For this review, use the dimensioned drawing (mm, ordinates from the lowest corner) and the shaded views. A direction names the side the tool comes from. Coordinates: 2 decimals unless noted, no trailing zeros. Order: outer loops, then holes, each group sorted by start corner. A loop starts at its lowest first (then second) coordinate and runs counter-clockwise, first axis right, second up. Notation, with made-up numbers: M 44.5,-21.75 L 55.5,-21.75 A15 ccw 55.5,-9.75 Z; hole C -28.5,-24.75 d7. An arc over 180 degrees is marked long. Answer in a Markdown table with one row per item.
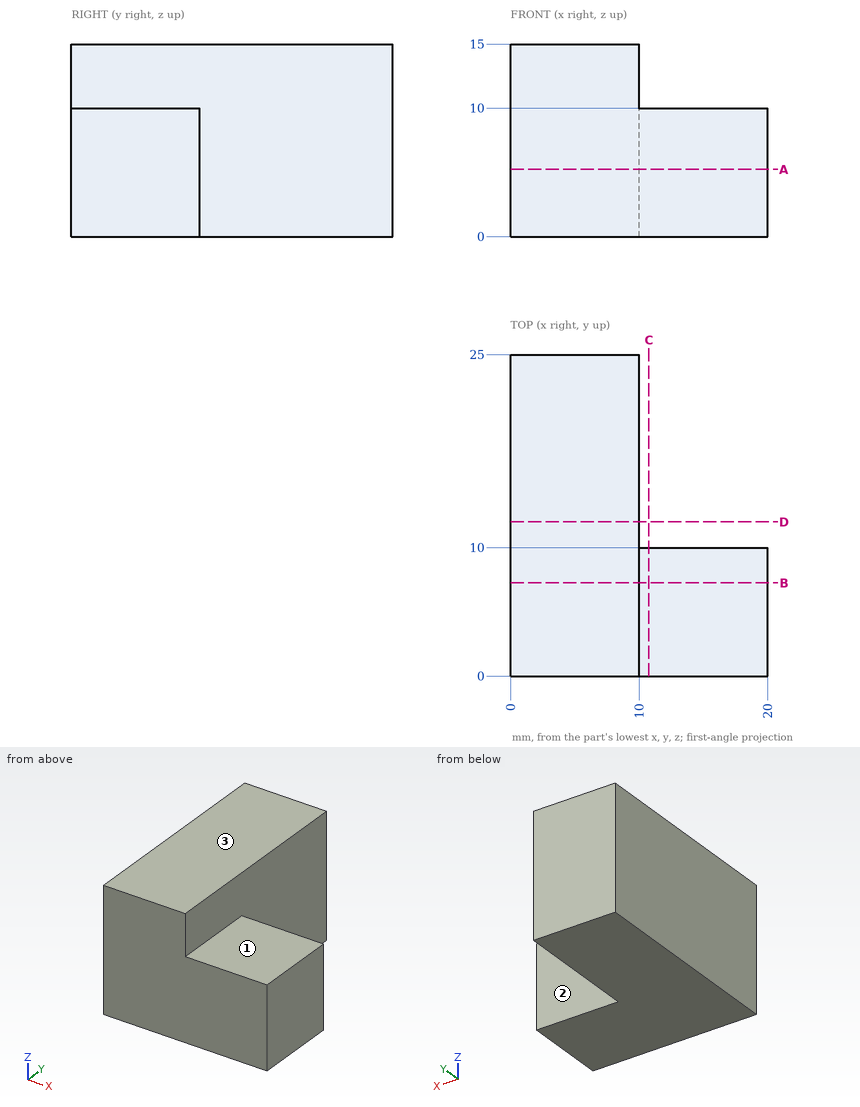
(1) Take a section at C-C (x = 10.75). Write out the cut boundary in (y, z).
Report:
| item | result |
|---|---|
| outline | M 0,0 L 10,0 L 10,10 L 0,10 Z |
(2) Take a section at D-D (y = 12). Write out the cut boundary in (x, z), then the cut area to 3 significant figures.
Report:
| item | result |
|---|---|
| outline | M 0,0 L 10,0 L 10,15 L 0,15 Z |
| area | 150 mm^2 |
(3) Take a section at A-A (z = 5.25). Write out the cut boundary in (x, y), then the cut area to 3 significant figures.
Report:
| item | result |
|---|---|
| outline | M 0,0 L 20,0 L 20,10 L 10,10 L 10,25 L 0,25 Z |
| area | 350 mm^2 |
(4) To check wall thickness, follow line 1 (X direction, y = 16.25, z = 2.25). State the ranges of the line that lie inside material, in increasing order. Write a range as [from, to].
Report:
| item | result |
|---|---|
| line 1 | [0, 10] |
(5) Insertion check: P1, Ø5, axis at x = 15, z = 8, coming from the +Y side; P2, Ø5, axis at x = 17.5, y = 5, coming from the +Z side. Each pin has a flat end and moves straight along its axis. Give the tip position at first contact, or say it passes through.
Report:
| item | result |
|---|---|
| P1 | y = 10 |
| P2 | z = 10 |
(6) Machinability: for the marked faces 1, 2 and 3, which of the approach directions +Z, -Z, +X, -X, +Y, -Y give a long, thin tool a straight path to every point of the face, cutting with its end or side? Answer none if there is none.
Report:
| item | result |
|---|---|
| face 1 | +Z, +X, +Y, -Y |
| face 2 | +Z, -Z, +X, +Y |
| face 3 | +Z, +X, -X, +Y, -Y |
(7) Take a section at B-B (y = 7.25). Write out the cut boundary in (x, z).
Report:
| item | result |
|---|---|
| outline | M 0,0 L 20,0 L 20,10 L 10,10 L 10,15 L 0,15 Z |
